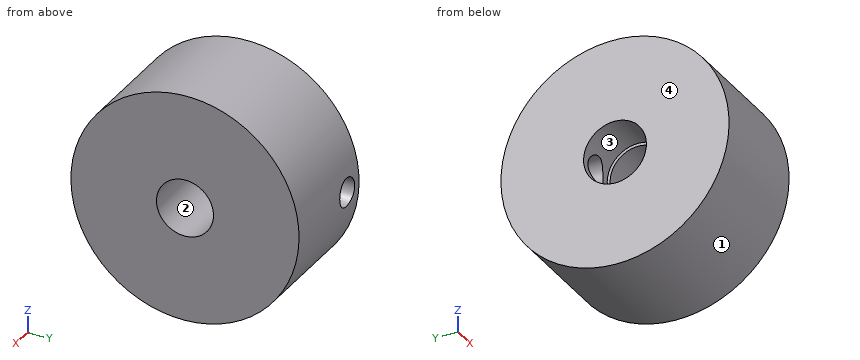
from build123d import *

# Parameters (mm, degrees)
SKETCH1_R                       = 12.7
BOSS_EXTRUDE1_DEPTH             = 12.7
SKETCH2_R                       = 3.5
CUT_EXTRUDE1_DEPTH              = 5
F_1_4_0_25_DIAMETER_HOLE1_D     = 6.35
F_1_4_0_25_DIAMETER_HOLE1_DEPTH = 10.16
F_1_4_0_25_DIAMETER_HOLE1_TIP   = 1.907732465


with BuildPart() as part:
    # Sketch1 → Boss-Extrude1 (new body)
    with BuildSketch(Plane(origin=(0, 0, 0), x_dir=(0, 0, -1), z_dir=(1, 0, 0))):
        Circle(SKETCH1_R)
    extrude(amount=BOSS_EXTRUDE1_DEPTH)

    # Sketch2 → Cut-Extrude1 (cut)
    with BuildSketch(Plane.ZY):
        Circle(SKETCH2_R)
    extrude(amount=-CUT_EXTRUDE1_DEPTH, mode=Mode.SUBTRACT)

    # 1/4 (0.25) Diameter Hole1
    with Locations(Plane(origin=(12.7, 0, 0), x_dir=(0, 0, -1), z_dir=(1, 0, 0))):
        with Locations((0, 0)):
            Hole(F_1_4_0_25_DIAMETER_HOLE1_D / 2, depth=F_1_4_0_25_DIAMETER_HOLE1_DEPTH)
            with Locations((0, 0, -(F_1_4_0_25_DIAMETER_HOLE1_DEPTH + F_1_4_0_25_DIAMETER_HOLE1_TIP / 2))):  # 118° drill point
                Cone(0, F_1_4_0_25_DIAMETER_HOLE1_D / 2, F_1_4_0_25_DIAMETER_HOLE1_TIP, mode=Mode.SUBTRACT)

    # Sketch7 → 1/8 (0.125) Diameter Hole1 (revolve, cut)
    with BuildSketch(Plane(origin=(2.5, 0, 0), x_dir=(0, 0, -1), z_dir=(1, 0, 0))):
        Polygon((0, 0), (0, 16.193866233), (1.5875, 15.24), (1.5875, 0), align=None)
    revolve(axis=Axis((2.5, -6.35, 0), (0, 1, 0)), mode=Mode.SUBTRACT)


solid = part.part
The model under review builds one solid part; all positions refer to its coordinate system, in mm. Face numbers are marked on the shaded views. Coordinates: 2 decimals unless noted, no trailing zeros. Loops run counter-clockwise (first coordinate to the right, second up) from the corner with the lowest first, then second, coordinate; pieces in that order, holes last. Notation, with made-up numbers: M 67,31 L 89,31 A15 cw 89,55 Z; hole C 33,-10.5 d6. An arc over 180 degrees is marked long. Put each result on its own line as item: value. Start each with the question number.
Q1. Add section C-C (z = -2.75). Write out the cut boundary in (x, y), and give its area (3 significant figures).
Q2. Add section A-A (y = 0). Write out the cut boundary in (x, z) (3 decimals), and give its area (3 significant figures).
Q3. Add section D-D (y = 9.5). Write out the cut boundary in (x, z) (1 decimal).
Q4. The part is to be moulded in two halves that separate along Y. For the marked faces 1, 2, 3 and 4, say which applies: +Y half, -Y half, draft (parallel to the pull), parting line (faces both ways), or undercut.
Q5. Add section B-B (z = 0). Count the separate pieces of the cut face and the enclosed holes in it, and give its area (3 significant figures).
Q6. Wall thickness on line 1 (Y direction, x = 10, z = 0) (3 decimals); line 2 (X direction, y = 5.5, z = 0); line 3 (X direction, y = 6.25, z = -0.75): over which ranges is each line inside the solid? List them lowest first.
Q7. Clearance check with flat-ended pins moving along their axes: pin 1 (6 mm diameter, centred on x = 8.5, y = 6, fed in from -Z); pin 2 (5 mm diameter, centred on x = 5, y = 8, fed in from -Z); pin 3 (5 mm diameter, centred on x = 7, z = 6.5, fed in from +Y); pin 4 (5 mm diameter, centred on y = 0, z = 0, fed in from -X). State where each tip first meets the part, or that it passes through.
Answers:
1. outline: M 0,-12.4 L 12.7,-12.4 L 12.7,-1.59 L 5,-1.59 L 5,-2.17 L 0,-2.17 Z; M 0,2.17 L 5,2.17 L 5,1.59 L 12.7,1.59 L 12.7,12.4 L 0,12.4 Z
1. area: 269 mm^2
2. outline: M 0,-12.7 L 12.7,-12.7 L 12.7,-3.175 L 5,-3.175 L 5,-3.5 L 0,-3.5 Z; M 0,3.5 L 5,3.5 L 5,3.175 L 12.7,3.175 L 12.7,12.7 L 0,12.7 Z
2. area: 239 mm^2
3. outline: M 0,-8.4 L 12.7,-8.4 L 12.7,8.4 L 0,8.4 Z; hole C 2.5,0 d3.2
4. face 1: parting line
4. face 2: undercut
4. face 3: undercut
4. face 4: draft
5. separate pieces: 3
5. enclosed holes: 0
5. area: 209 mm^2
6. line 1: y = -12.7 to -3.175, 3.175 to 12.7
6. line 2: x = 0 to 0.91, 4.09 to 12.7
6. line 3: x = 0 to 1.1, 3.9 to 12.7
7. pin 1: stops at z = -12.34
7. pin 2: stops at z = -11.45
7. pin 3: stops at y = 12.05
7. pin 4: passes through
